For this review, take the finished solid that the model builds, in its own axes (mm). Give positions to 0.01 mm unless a question says otherwise; leave off trailing zeros. Write each loop counter-clockwise with the first axis right and the second up, starting at its lowest first coordinate (ties: lowest second). Pieces come first, ordered by that corner, then holes. Notation, with made-up numbers: M 20,77 L 43,77 A20 cw 43,90 Z; hole C 57.25,40 d3. An arc over 180 degrees is marked long. Write item = value, one per line.
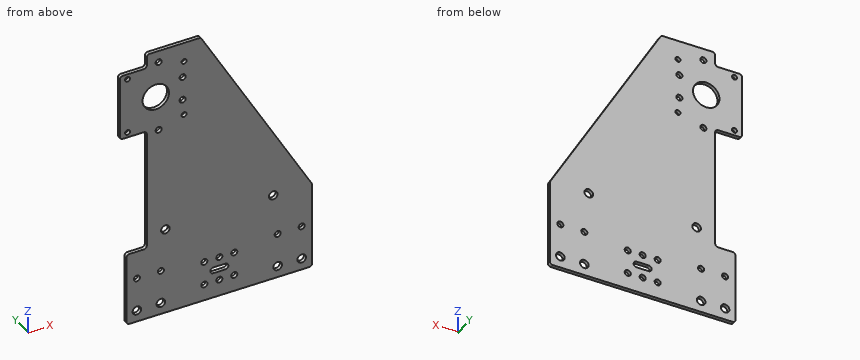
```python
from build123d import *

# Parameters (mm, degrees)
F0_W     = 10
F0_H     = 5.1
F1_DEPTH = 3
F2_D     = 22
F3_D     = 4.2
F4_D     = 5.1
F5_D     = 7.2


with BuildPart() as f1:
    # F0 (on Front) → F1 (new body)
    with BuildSketch(Plane.XZ):
        with BuildLine():
            ThreePointArc((-58, 210), (-59.767766953, 209.267766953), (-60.5, 207.5))
            Line((-60.5, 207.5), (-60.5, 200.5))
            ThreePointArc((-60.5, 200.5), (-61.232233047, 198.732233047), (-63, 198))
            Line((-63, 198), (-80.5, 198))
            ThreePointArc((-80.5, 198), (-82.267766953, 197.267766953), (-83, 195.5))
            Line((-83, 195.5), (-83, 144.5))
            ThreePointArc((-83, 144.5), (-82.267766953, 142.732233047), (-80.5, 142))
            Line((-80.5, 142), (-63, 142))
            ThreePointArc((-63, 142), (-61.232233047, 141.267766953), (-60.5, 139.5))
            Line((-60.5, 139.5), (-60.5, 40.5))
            ThreePointArc((-60.5, 40.5), (-61.232233047, 38.732233047), (-63, 38))
            Line((-63, 38), (-75, 38))
            ThreePointArc((-75, 38), (-76.767766953, 37.267766953), (-77.5, 35.5))
            Line((-77.5, 35.5), (-77.5, -21.5))
            ThreePointArc((-77.5, -21.5), (-76.767766953, -23.267766953), (-75, -24))
            Line((-75, -24), (75, -24))
            ThreePointArc((75, -24), (76.767766953, -23.267766953), (77.5, -21.5))
            Line((77.5, -21.5), (77.5, 48.3298361723))
            ThreePointArc((77.5, 48.3298361723), (77.4147443195, 48.9771458907), (77.1647921028, 49.5803061447))
            Line((77.1647921028, 49.5803061447), (-14.7782217853, 208.7504699724))
            ThreePointArc((-14.7782217853, 208.7504699724), (-15.6932488963, 209.6651991746), (-16.943013888, 210))
            Line((-16.943013888, 210), (-58, 210))
        make_face()
        Rectangle(F0_W, F0_H, mode=Mode.SUBTRACT)
    extrude(amount=F1_DEPTH)

    # F2 (through all)
    with Locations(Plane(origin=(0, 0, 0), x_dir=(1, 0, 0), z_dir=(0, 1, 0))):
        with Locations((-53, -170)):
            Hole(F2_D / 2)

    # F3 (through all)
    with Locations(Plane(origin=(0, 0, 0), x_dir=(1, 0, 0), z_dir=(0, 1, 0))):
        with Locations((-76.57, -193.57), (-29.43, -193.57), (-29.43, -146.43), (-76.57, -146.43)):
            Hole(F3_D / 2)

    # F4 (through all)
    with Locations(Plane(origin=(0, 0, 0), x_dir=(1, 0, 0), z_dir=(0, 1, 0))):
        with Locations((-50.6, -200), (-30.6, -180), (-30.6, -160), (-50.6, -140), (-68.74, -14.25), (-48.74, -14.25), (48.74, -14.25), (68.74, -14.25), (12.5, -10), (0, -10), (-12.5, -10), (-12.5, 10), (0, 10), (12.5, 10), (5, 0), (-5, 0)):
            Hole(F4_D / 2)

    # F5 (through all)
    with Locations(Plane(origin=(0, 0, 0), x_dir=(1, 0, 0), z_dir=(0, 1, 0))):
        with Locations((-68.74, 14.25), (-48.74, 14.25), (48.74, 14.25), (68.74, 14.25), (-45, -49.75), (45, -49.75)):
            Hole(F5_D / 2)


solid = f1.part
```
1. We need section B-B, the plane x = -12.5. Write out the cut boundary in (y, z).
Responses:
outline = M -3,-24 L 0,-24 L 0,-12.55 L -3,-12.55 Z; M -3,-7.45 L 0,-7.45 L 0,7.45 L -3,7.45 Z; M -3,12.55 L 0,12.55 L 0,204.81 L -3,204.81 Z
2. For line 1 along X through (y, z) = (-1.1, -14.25); line 2 along Z through (x, y) = (-68.74, -1.85); line 3 along X through (y, z) = (-0.8, 14.25), list the stretches that pass through material, from the lowest coordinate up. Write a range as from..to.
Responses:
line_1 = -77.5..-72.34, -65.14..-52.34, -45.14..45.14, 52.34..65.14, 72.34..77.5
line_2 = -24..-17.85, -10.65..11.7, 16.8..38, 142..198
line_3 = -77.5..-71.29, -66.19..-51.29, -46.19..46.19, 51.29..66.19, 71.29..77.5
3. We need section A-A, the plane z = 0. Write out the cut boundary in (x, y), then the cut area to 3 significant figures.
Responses:
outline = M -77.5,-3 L -7.55,-3 L -7.55,0 L -77.5,0 Z; M 7.55,-3 L 77.5,-3 L 77.5,0 L 7.55,0 Z
area = 420 mm2
4. We need section D-D, the plane z = 170. Write out the cut boundary in (x, y).
Responses:
outline = M -83,-3 L -64,-3 L -64,0 L -83,0 Z; M -42,-3 L 7.61,-3 L 7.61,0 L -42,0 Z
5. We need section C-C, the plane y = -1.9. Count the separate pieces of the cut face and the enclosed holes in it, then the cut area to 3 significant figures.
Responses:
separate_pieces = 1
enclosed_holes = 26
area = 26,100 mm2
6. Insertion check: P1, Ø1.5, axis at y = -2, z = 32, coming from the -X side. The pin has a flat end and moves straight along its axis. Give the tip position at first contact, or say it passes through.
Responses:
P1 = -77.5
